from build123d import *

# Parameters (mm, degrees)
SKETCH_1_W          = 2
SKETCH_1_H          = 9
SKETCH_2_W          = 1
SKETCH_2_H          = 1
CUT_EXTRUDE_1_DEPTH = 10
CHAMFER_1_SIZE      = 1.5


with BuildPart() as part:
    # Эскиз1 → Повернуть1 (revolve)
    with BuildSketch(Plane.XY):
        with Locations((-1, 7.5)):
            Rectangle(SKETCH_1_W, SKETCH_1_H)
        Polygon((-4, 0), (0, 0), (0, 3), (-2, 3), (-4, 1), align=None)
    revolve(axis=Axis((0, 12, 0), (0, -1, 0)))

    # Эскиз2 → Вырез-Вытянуть1 (cut, symmetric)
    with BuildSketch(Plane.XY):
        with Locations((0, 0.5)):
            Rectangle(SKETCH_2_W, SKETCH_2_H)
    extrude(amount=CUT_EXTRUDE_1_DEPTH, both=True, mode=Mode.SUBTRACT)

    # Фаска1
    chamfer_1_edges = [part.edges().sort_by_distance(p)[0] for p in [
        (2, 12, 0),
    ]]
    chamfer(chamfer_1_edges, length=CHAMFER_1_SIZE)


solid = part.part
Geometry check sheet. Reference: the model listing, model coordinates, mm. A direction names the side the tool comes from. Give positions to 0.01 mm unless a question says otherwise; leave off trailing zeros. Order: outer loops, then holes, each group sorted by start corner. A loop starts at its lowest first (then second) coordinate and runs counter-clockwise, first axis right, second up.
1) Tool access check on faces 1 (the cylindrical face through (0, 7, 2)), 2 (the flat face through (0.5, 0.5, 0.1)), 3 (the flat face through (0, 12, 0)). Record the directions out of +Z, -Z, +X, -X, +Y, -Y that give a thin tool (end or side, any length) a straight path to the whole face; none if there is none.
Results are:
face 1: +Y
face 2: +Z, -Z, -Y
face 3: +Z, -Z, +X, -X, +Y
2) Cross-section at C-C (z = 0). Record the boundary of the cut face in (x, y), then the cut area to 4 significant figures.
Results are:
outline: (-4, 0) - (-0.5, 0) - (-0.5, 1) - (0.5, 1) - (0.5, 0) - (4, 0) - (4, 1) - (2, 3) - (2, 10.5) - (0.5, 12) - (-0.5, 12) - (-2, 10.5) - (-2, 3) - (-4, 1) - close
area: 52.75 mm2
3) Cross-section at A-A (x = 0). Record the boundary of the cut face in (y, z), then the cut area to 4 significant figures.
Results are:
outline: (1, -4) - (3, -2) - (10.5, -2) - (12, -0.5) - (12, 0.5) - (10.5, 2) - (3, 2) - (1, 4) - close
area: 45.75 mm2
4) Gauge pin test, flat ends, axial feed: pin 1 (0.5 mm diameter, centred on y = 0.5, z = 1.5, fed in from +X); pin 2 (0.8 mm diameter, centred on x = 0, z = 1.5, fed in from -Y); pin 3 (1.5 mm diameter, centred on x = 2, y = 6, fed in from +Z). Record the tip position at first contact, or that the pin passes through.
Results are:
pin 1: stops at x = 3.8
pin 2: stops at y = 1
pin 3: stops at z = 1.56
5) Draft check along X on faces 4 (the flat face through (-0.5, 0.5, 0.1)), 5 (the flat face through (2, 0, 0)), 6 (the flat face through (0, 1, 0)), 7 (the cylindrical face through (4, 0.5, -0.1)). Enter one of: released by +X, released by -X, zero draft, split by the parting line, or undercut.
Results are:
face 4: undercut
face 5: zero draft
face 6: undercut
face 7: released by +X
6) Cross-section at B-B (y = 0.5). Record the boundary of the cut face in (x, z).
Results are:
outline: (-0.5, -3.97) - (-0.5, 3.97) arc R4 ccw to start; (0.5, -3.97) arc R4 ccw to (0.5, 3.97) - close
7) Cross-section at D-D (y = 7). Record the boundary of the cut face in (x, z), then the cut area to 3 significant figures.
Results are:
outline: circle Ø4 at (0, 0)
area: 12.6 mm2
8) Material ranges on probe 1 along X at (y, z) = (4.5, 0); probe 2 along Y at (x, z) = (2, -2); probe 3 along Y at (x, z) = (2, -0.75), recorded low to high.
Results are:
probe 1: x = -2 to 2
probe 2: y = 0 to 2.17
probe 3: y = 0 to 2.86
